Verification items for the finished model (mm, model axes). Face numbers are marked on the shaded views. A direction names the side the tool comes from. Coordinates: 2 decimals unless noted, no trailing zeros. Order: outer loops, then holes, each group sorted by start corner. A loop starts at its lowest first (then second) coordinate and runs counter-clockwise, first axis right, second up. Notation, with made-up numbers: M 12,18.25 L 28,18.25 A27 ccw 28,48.25 Z; hole C -33,74 d7. An arc over 180 degrees is marked long. Return JSON: item names as keys, results as strings. Group by question number.
Q1. Section check D-D, the plane x = 20. Enter the section's corners in (y, z), then the cut area to 3 significant figures.
Q2. Mould release check, pull along Z, two halves, no side actions. Record for the marked faces 1, 2, 3 and 4: pulls with the +Z half, pulls with the -Z half, needs draft (parallel to the pull), parting line crosses it, or undercut.
Q3. Section check A-A, the plane z = -4.5. Enter the section's corners in (x, y).
Q4. Section check C-C, the plane x = 35. Enter the section's corners in (y, z), then the cut area to 3 significant figures.
Q5. Section check B-B, the plane y = 16. Enter the section's corners in (x, z), then the cut area to 3 significant figures.
Q6. Go/stop test with flat-tipped pins: pin 1 Ø1.5 at (x, y) = (17, 21.5) entering from +Z; pin 2 Ø1.5 at (x, z) = (10.5, -3.5) entering from +Y; pin 3 Ø0.8 at (y, z) = (10, -8.5) entering from +X. Record where each tip stops, or that it passes through.
Q7. Thickness scan on probe 1 along Z at (x, y) = (18, 1.75); probe 2 along Z at (x, y) = (5, 0.7); probe 3 along Y at (x, z) = (24.5, -8.25). Record the ranges inside material, lowest first.
Q8. Access from +Z, -Z, +X, -X, +Y, -Y to the whole of each face (thin tool, end or side, straight path). Record for the marked faces 5 and 6.
from build123d import *

# Parameters (mm, degrees)
SKETCH_1_W                = 40
SKETCH_1_H                = 9
SKETCH_1_W_2              = 15
SKETCH_1_H_2              = 7
EXTRUDE_1_DEPTH           = 1
SKETCH_2_W                = 20
SKETCH_2_H                = 20
SKETCH_2_R                = 1.5
EXTRUDE_2_DEPTH           = 1
EXTRUDE_START             = -8
SKETCH_2_2_W              = 20
SKETCH_2_2_H              = 20
SKETCH_2_2_R              = 1.5
EXTRUDE_3_DEPTH           = 1
HOLE_WIZARD_5_0_5_1_D     = 5
HOLE_WIZARD_5_0_5_1_DEPTH = 6
EXTRUDE_START_2           = 7
SKETCH_5_R                = 7
SKETCH_5_R_2              = 1.5
EXTRUDE_4_DEPTH           = 7
FILLET_1_R                = 3


with BuildPart() as part:
    # 草图1 → 凸台-拉伸1 (new body)
    with BuildSketch(Plane(origin=(0, 0, 0), x_dir=(1, 0, 0), z_dir=(0, 1, 0))):
        with Locations((20, 4.5)):
            Rectangle(SKETCH_1_W, SKETCH_1_H)
        with Locations((20, 4.5)):
            Rectangle(SKETCH_1_W_2, SKETCH_1_H_2, mode=Mode.SUBTRACT)
    extrude(amount=EXTRUDE_1_DEPTH)

    # 草图2 → 凸台-拉伸2 (add)
    with BuildSketch(Plane.XY):
        with Locations((20, 10)):
            Rectangle(SKETCH_2_W, SKETCH_2_H)
        with Locations((20, 16)):
            Circle(SKETCH_2_R, mode=Mode.SUBTRACT)
    extrude(amount=-EXTRUDE_2_DEPTH)

    # 草图2<2> → 凸台-拉伸3 (add)
    with BuildSketch(Plane.XY.offset(EXTRUDE_START)):
        with Locations((20, 10)):
            Rectangle(SKETCH_2_2_W, SKETCH_2_2_H)
        with Locations((20, 16)):
            Circle(SKETCH_2_2_R, mode=Mode.SUBTRACT)
    extrude(amount=-EXTRUDE_3_DEPTH)

    # Ø5.0 (5) 直径孔1
    with Locations(Plane(origin=(0, 1, 0), x_dir=(1, 0, 0), z_dir=(0, 1, 0))):
        with Locations((35, 4.5), (5, 4.5)):
            Hole(HOLE_WIZARD_5_0_5_1_D / 2, depth=HOLE_WIZARD_5_0_5_1_DEPTH)

    # 草图5 → 凸台-拉伸4 (add)
    with BuildSketch(Plane.XY.offset(-8).offset(EXTRUDE_START_2)):
        with Locations(Location((20, 16, 0), (0, 0, 145.150095421))):
            Circle(SKETCH_5_R)
        with Locations((20, 16)):
            Circle(SKETCH_5_R_2, mode=Mode.SUBTRACT)
    extrude(amount=-EXTRUDE_4_DEPTH)

    # 圆角1
    fillet_1_edges = [part.edges().sort_by_distance(p)[0] for p in [
        (30, 20, -0.5),
        (10, 20, -0.5),
        (10, 20, -8.5),
        (30, 20, -8.5),
        (0, 0.5, -9),
        (40, 0.5, -9),
        (40, 0.5, 0),
        (0, 0.5, 0),
    ]]
    fillet(fillet_1_edges, radius=FILLET_1_R)


solid = part.part
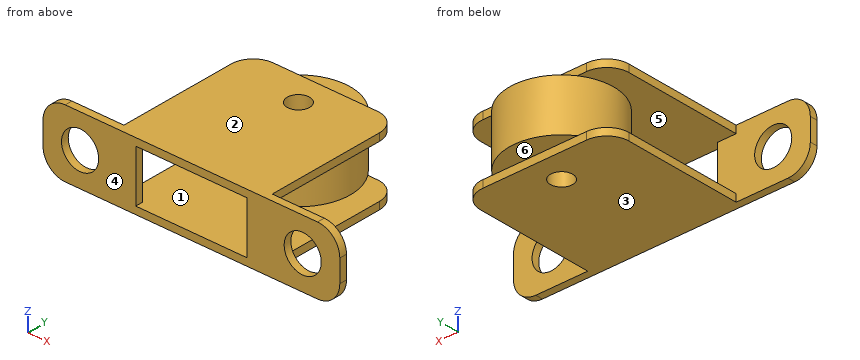
Numbers:
{
 "1": {"outline": "M 0,-9 L 14.5,-9 L 14.5,0 L 0,0 L 0,-1 L 9,-1 L 9,-8 L 0,-8 Z; M 17.5,-9 L 20,-9 L 20,-8 L 23,-8 L 23,-1 L 20,-1 L 20,0 L 17.5,0 Z", "area": "111 mm2"},
 "2": {"face 1": "undercut", "face 2": "pulls with the +Z half", "face 3": "pulls with the -Z half", "face 4": "needs draft"},
 "3": {"outline": "M 0,0 L 2.5,0 L 2.5,1 L 0,1 Z; M 7.5,0 L 12.5,0 L 12.5,1 L 7.5,1 Z; C 20,16 d14; M 27.5,0 L 32.5,0 L 32.5,1 L 27.5,1 Z; M 37.5,0 L 40,0 L 40,1 L 37.5,1 Z; hole C 20,16 d3"},
 "4": {"outline": "M 0,-9 L 1,-9 L 1,-7 L 0,-7 Z; M 0,-2 L 1,-2 L 1,0 L 0,0 Z", "area": "4.00 mm2"},
 "5": {"outline": "M 10,-9 L 18.5,-9 L 18.5,0 L 10,0 L 10,-1 L 13,-1 L 13,-8 L 10,-8 Z; M 21.5,-9 L 30,-9 L 30,-8 L 27,-8 L 27,-1 L 30,-1 L 30,0 L 21.5,0 Z", "area": "111 mm2"},
 "6": {"pin 1": "stops at z = -1", "pin 2": "stops at y = 1", "pin 3": "stops at x = 30"},
 "7": {"probe 1": "z = -9 to -8, -1 to 0", "probe 2": "z = -9 to -7, -2 to 0", "probe 3": "y = 0 to 20"},
 "8": {"face 5": "none", "face 6": "-Z, +X, -X, +Y"}
}
